Work out the finished part from the listing and answer in its coordinate system (mm). Face numbers are marked on the shaded views. A direction names the side the tool comes from. Round coordinates to 2 decimals unless told otherwise and drop trailing zeros. Write each loop counter-clockwise with the first axis right and the second up, starting at its lowest first coordinate (ties: lowest second). Pieces come first, ordered by that corner, then holes. Notation, with made-up numbers: (71, -23.75) -> (118, -23.75) arc R19 cw to (118, 4.25) -> close; hole circle Ø11 at (14.25, 57.25). An arc over 180 degrees is marked (long way). One line per item, written item: value.
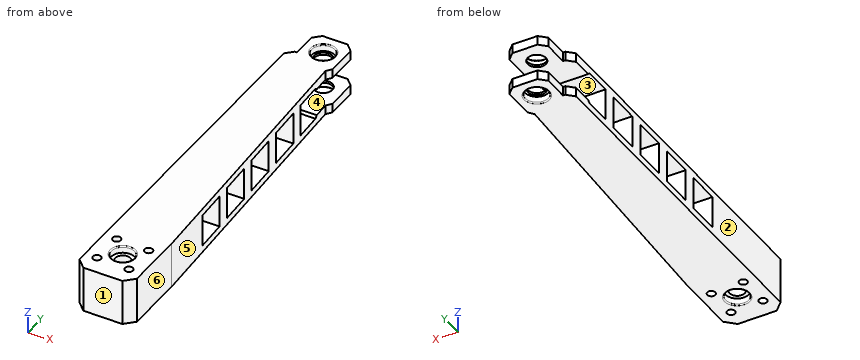
```python
from build123d import *
from OCP.BRepFilletAPI import BRepFilletAPI_MakeChamfer

# Parameters (mm, degrees)
SKETCH_1_R          = 1.75
EXTRUDE_1_DEPTH     = 20
CHAMFER_1_SIZE      = 4
SKETCH_2_R          = 5.05
CUT_EXTRUDE_1_DEPTH = 3
SKETCH_3_R          = 3.3
CUT_EXTRUDE_2_DEPTH = 32
CUT_EXTRUDE_START   = -3
SKETCH_4_R          = 5.05
CUT_EXTRUDE_3_DEPTH = 3
CHAMFER_2_SIZE      = 3
CHAMFER_2_SIZE2     = 3.148509384
SKETCH_6_W          = 14
SKETCH_6_H          = 14
CUT_EXTRUDE_4_DEPTH = 58
EXTRUDE_2_DEPTH     = 4
SKETCH_8_R          = 5.05
CUT_EXTRUDE_5_DEPTH = 3
SKETCH_9_R          = 4
CUT_EXTRUDE_6_DEPTH = 3
CHAMFER_3_SIZE      = 3
CHAMFER_4_SIZE      = 3
CHAMFER_5_SIZE      = 2
FILLET_1_R          = 0.5
FILLET_2_R          = 0.5
FILLET_3_R          = 0.5


with BuildPart() as part:
    # 草图1 → 凸台-拉伸1 (new body)
    with BuildSketch(Plane.XY):
        Polygon((12.5, -50), (6.5, 80), (-12.5, 80), (-12.5, -80), (12.5, -80), align=None)
        with Locations((-6.881060168, -57.743898363)):
            Circle(SKETCH_1_R, mode=Mode.SUBTRACT)
        with Locations((7.256101637, -58.118939832)):
            Circle(SKETCH_1_R, mode=Mode.SUBTRACT)
        with Locations((6.881060168, -72.256101637)):
            Circle(SKETCH_1_R, mode=Mode.SUBTRACT)
        with Locations((-7.256101637, -71.881060168)):
            Circle(SKETCH_1_R, mode=Mode.SUBTRACT)
    extrude(amount=EXTRUDE_1_DEPTH)

    # 倒角1
    chamfer_1_edges = [part.edges().sort_by_distance(p)[0] for p in [
        (12.5, -80, 10),
        (-12.5, -80, 10),
    ]]
    chamfer(chamfer_1_edges, length=CHAMFER_1_SIZE)

    # 草图2 → 切除-拉伸1 (cut)
    with BuildSketch(Plane.XY.offset(20)):
        with Locations((0, -65)):
            Circle(SKETCH_2_R)
    extrude(amount=-CUT_EXTRUDE_1_DEPTH, mode=Mode.SUBTRACT)

    # 草图3 → 切除-拉伸2 (cut)
    with BuildSketch(Plane(origin=(0, 0, 0), x_dir=(-1, 0, 0), z_dir=(0, 0, -1))):
        with Locations((0, -65)):
            Circle(SKETCH_3_R)
    extrude(amount=-CUT_EXTRUDE_2_DEPTH, mode=Mode.SUBTRACT)

    # 草图4 → 切除-拉伸3 (cut)
    with BuildSketch(Plane(origin=(0, 0, 0), x_dir=(-1, 0, 0), z_dir=(0, 0, -1)).offset(CUT_EXTRUDE_START)):
        with Locations(Location((0, -65, 0), (0, 0, 180))):
            Circle(SKETCH_4_R)
    extrude(amount=CUT_EXTRUDE_3_DEPTH, mode=Mode.SUBTRACT)

    # 倒角2: one chamfer whose edges measure the first distance from different faces: ONE call of the kernel's chamfer builder (chamfer() names one face for all edges)
    chamfer_2_edges_1 = [part.edges().sort_by_distance(p)[0] for p in [
        (-12.5, 80, 10),
    ]]
    chamfer_2_edges_2 = [part.edges().sort_by_distance(p)[0] for p in [
        (6.5, 80, 10),
    ]]
    chamfer_2_side_2 = [part.faces().sort_by_distance(p)[0] for p in [
        (9.5, 15, 10),
    ]]
    chamfer_2 = BRepFilletAPI_MakeChamfer(part.part.solid().wrapped)
    for e in chamfer_2_edges_1:
        chamfer_2.Add(CHAMFER_2_SIZE, e.wrapped)
    for e in chamfer_2_edges_2:
        chamfer_2.Add(CHAMFER_2_SIZE, CHAMFER_2_SIZE2, e.wrapped, chamfer_2_side_2[0].wrapped)  # the first distance lies on this face
    add(Compound.cast(chamfer_2.Shape()), mode=Mode.REPLACE)

    # 草图6 → 切除-拉伸4 (cut)
    with BuildSketch(Plane.ZY.offset(12.5)):
        Polygon((3, 69), (4, 69), (4, 86.606833076), (16, 86.606833076), (16, 69), (17, 69), (17, 55), (3, 55), align=None)
        with Locations((10, 42)):
            Rectangle(SKETCH_6_W, SKETCH_6_H)
        with Locations((10, 22)):
            Rectangle(SKETCH_6_W, SKETCH_6_H)
        with Locations((10, 2)):
            Rectangle(SKETCH_6_W, SKETCH_6_H)
        with Locations((10, -18)):
            Rectangle(SKETCH_6_W, SKETCH_6_H)
    extrude(amount=-CUT_EXTRUDE_4_DEPTH, mode=Mode.SUBTRACT)

    # 草图7 → 凸台-拉伸2 (add)
    with BuildSketch(Plane(origin=(0, 0, 0), x_dir=(-1, 0, 0), z_dir=(0, 0, -1))):
        Polygon((8.5, 93.975326294), (-4.475326294, 93.975326294), (-6.6383143, 93.975326294), (-8.4383143, 93.975326294), (-8.4383143, 77.287576761), (-6.730769231, 75), (-6.6383143, 77.00319017), (-4.475326294, 78.975326294), (-3.351490616, 80), (8.5, 80), align=None)
    extrude_2 = extrude(amount=-EXTRUDE_2_DEPTH)

    # 镜向1: 凸台-拉伸2 across plane
    add(extrude_2.mirror(Plane.XY.offset(10)))

    # 草图8 → 切除-拉伸5 (cut)
    with BuildSketch(Plane(origin=(0, 0, 0), x_dir=(-1, 0, 0), z_dir=(0, 0, -1))):
        with Locations((0, 85)):
            Circle(SKETCH_8_R)
    cut_extrude_5 = extrude(amount=-CUT_EXTRUDE_5_DEPTH, mode=Mode.SUBTRACT)

    # 草图9 → 切除-拉伸6 (cut)
    with BuildSketch(Plane(origin=(0, 0, 3), x_dir=(-1, 0, 0), z_dir=(0, 0, -1))):
        with Locations((0, 85)):
            Circle(SKETCH_9_R)
    cut_extrude_6 = extrude(amount=-CUT_EXTRUDE_6_DEPTH, mode=Mode.SUBTRACT)

    # 镜向2: 切除-拉伸5, 切除-拉伸6 across plane
    add(cut_extrude_5.mirror(Plane.XY.offset(10)), mode=Mode.SUBTRACT)
    add(cut_extrude_6.mirror(Plane.XY.offset(10)), mode=Mode.SUBTRACT)

    # 倒角3
    chamfer_3_edges = [part.edges().sort_by_distance(p)[0] for p in [
        (8.4383143, 93.975326294, 2),
        (-8.5, 93.975326294, 2),
    ]]
    chamfer(chamfer_3_edges, length=CHAMFER_3_SIZE)

    # 倒角4
    chamfer_4_edges = [part.edges().sort_by_distance(p)[0] for p in [
        (-8.5, 93.975326294, 18),
        (8.4383143, 93.975326294, 18),
    ]]
    chamfer(chamfer_4_edges, length=CHAMFER_4_SIZE)

    # 倒角5
    # the kernel refuses this chamfer: 2 mm, written as the material it adds along each edge
    with BuildSketch(Plane(origin=(-12.5, 69, 3), x_dir=(0, -0.9996219169112968, -0.0274958766105862), z_dir=(1, 0, 0))) as chamfer_5_piece_1_section:
        Polygon((CHAMFER_5_SIZE * 0.999621916911, -CHAMFER_5_SIZE * 0.0274958766106), (-CHAMFER_5_SIZE * 0.0274958766106, -CHAMFER_5_SIZE * 0.999621916911), (0, 0), align=None)
    chamfer_5_piece_1 = extrude(amount=24.651058284, mode=Mode.PRIVATE)
    chamfer_5_piece_1 = split(chamfer_5_piece_1, bisect_by=Plane(origin=(7.023262374, 68.662648572, 3.416350106), z_dir=(-0.9989366098486855, -0.04610476660840088, 0)), keep=Keep.TOP, mode=Mode.PRIVATE)
    chamfer_5_piece_1 = split(chamfer_5_piece_1, bisect_by=Plane(origin=(-2.727982872, 68.212591099, 4), z_dir=(0, 0, -1)), keep=Keep.TOP, mode=Mode.PRIVATE)
    add(chamfer_5_piece_1)
    with BuildSketch(Plane(origin=(-12.5, 69, 17), x_dir=(0, 0.02749587661058907, -0.9996219169112965), z_dir=(1, 0, 0))) as chamfer_5_piece_2_section:
        Polygon((CHAMFER_5_SIZE * 0.999621916911, -CHAMFER_5_SIZE * 0.0274958766106), (-CHAMFER_5_SIZE * 0.0274958766106, -CHAMFER_5_SIZE * 0.999621916911), (0, 0), align=None)
    chamfer_5_piece_2 = extrude(amount=24.651058284, mode=Mode.PRIVATE)
    chamfer_5_piece_2 = split(chamfer_5_piece_2, bisect_by=Plane(origin=(7.023262374, 68.662648572, 16.583649894), z_dir=(-0.9989366098486855, -0.04610476660840088, 0)), keep=Keep.TOP, mode=Mode.PRIVATE)
    chamfer_5_piece_2 = split(chamfer_5_piece_2, bisect_by=Plane(origin=(-2.727982872, 68.212591099, 16), z_dir=(0, 0, 1)), keep=Keep.TOP, mode=Mode.PRIVATE)
    add(chamfer_5_piece_2)

    # 圆角1
    fillet_1_edges = [part.edges().sort_by_distance(p)[0] for p in [
        (-5.05, -65, 0),
    ]]
    fillet(fillet_1_edges, radius=FILLET_1_R)

    # 圆角2
    fillet_2_edges = [part.edges().sort_by_distance(p)[0] for p in [
        (-5.05, -65, 20),
    ]]
    fillet(fillet_2_edges, radius=FILLET_2_R)

    # 圆角3
    fillet_3_edges = [part.edges().sort_by_distance(p)[0] for p in [
        (5.05, 85, 0),
        (5.05, 85, 20),
    ]]
    fillet(fillet_3_edges, radius=FILLET_3_R)


solid = part.part
```
(1) Find section B-B on z = 11.75. Give the number of separate pieces and of enclosed holes in the cut face, plus the area to 3 significant figures.
Reported:
separate pieces: 5
enclosed holes: 5
area: 1,790 mm2
(2) Find section A-A on y = -65. Give the vertices of the cut face in (x, z), plus the area to 3 significant figures.
Reported:
outline: (-12.5, 0) -> (-5.55, 0) arc R0.5 ccw to (-5.05, 0.5) -> (-5.05, 3) -> (-3.3, 3) -> (-3.3, 17) -> (-5.05, 17) -> (-5.05, 19.5) arc R0.5 ccw to (-5.55, 20) -> (-12.5, 20) -> close; (3.3, 3) -> (5.05, 3) -> (5.05, 0.5) arc R0.5 ccw to (5.55, 0) -> (12.5, 0) -> (12.5, 20) -> (5.55, 20) arc R0.5 ccw to (5.05, 19.5) -> (5.05, 17) -> (3.3, 17) -> close
area: 347 mm2
(3) A tool of negligible diameter and unlimited length cuts with its end or side. For the marked faces 4, 5 and 6, from which of +Z, -Z, +X, -X, +Y, -Y can it reach the whole face along a straight path? Write none if from no direction.
Reported:
face 4: +X, -X, +Y
face 5: +Z, -Z, +X
face 6: +Z, -Z, +X, +Y, -Y
(4) For a pull along Y with two mould halves and no side action, classify the marked faces 1, 2 and 3 as pulls with the +Y half, pulls with the -Y half, needs draft (parallel to the pull), parting line crosses it, or undercut.
Reported:
face 1: pulls with the -Y half
face 2: needs draft
face 3: undercut
(5) Consider probe 1 along Y at (x, z) = (0, 18.65); probe 2 along Y at (x, z) = (3.5, 12.25); probe 3 along X at (y, z) = (85, 16.7). Determine where each line is inside the solid, lowest interval first.
Reported:
probe 1: y = -80 to -70.05, -59.95 to 79.95, 90.05 to 93.98
probe 2: y = -80 to -25, -11 to -5, 9 to 15, 29 to 35, 49 to 55
probe 3: x = -8.5 to -4, 4 to 8.44
(6) Flat-ended cylindrical pins translate along their axes: pin 1 Ø11 at (x, y) = (0.5, 43.5) entering from -Z; pin 2 Ø4 at (y, z) = (-19.5, 17.5) entering from +X; pin 3 Ø1 at (x, z) = (3, 5) entering from +Y; pin 4 Ø3 at (y, z) = (83, 1) entering from -X. Find the tip coordinate at first contact, or state that the pin passes through.
Reported:
pin 1: stops at z = 0
pin 2: stops at x = 11.18
pin 3: stops at y = 55
pin 4: stops at x = -8.5
(7) Find section C-C on y = 85. Give the vertices of the cut face in (x, z), plus the area to 3 significant figures.
Reported:
outline: (-8.5, 0) -> (-5.55, 0) arc R0.5 ccw to (-5.05, 0.5) -> (-5.05, 3) -> (-4, 3) -> (-4, 4) -> (-8.5, 4) -> close; (-8.5, 16) -> (-4, 16) -> (-4, 17) -> (-5.05, 17) -> (-5.05, 19.5) arc R0.5 ccw to (-5.55, 20) -> (-8.5, 20) -> close; (4, 3) -> (5.05, 3) -> (5.05, 0.5) arc R0.5 ccw to (5.55, 0) -> (8.44, 0) -> (8.44, 4) -> (4, 4) -> close; (4, 16) -> (8.44, 16) -> (8.44, 20) -> (5.55, 20) arc R0.5 ccw to (5.05, 19.5) -> (5.05, 17) -> (4, 17) -> close
area: 58.7 mm2
